CAD build for the part. Positions are in the model's coordinates, mm. A direction names the side the tool comes from. Coordinates: 2 decimals unless noted, no trailing zeros. Order: outer loops, then holes, each group sorted by start corner. A loop starts at its lowest first (then second) coordinate and runs counter-clockwise, first axis right, second up.
Autodesk Inventor part; units mm, degrees
ref_plane "Work Plane1" through (10.95, 0, 0) normal (0, 0, -1) x (1, 0, 0)
ref_plane "YZ Plane" through (0, 0, 0) normal (1, 0, 0) x (0, 1, 0)
ref_plane "XZ Plane" through (0, 0, 0) normal (0, 1, 0) x (-1, 0, 0)
sketch "Sketch1" plane through (0, 0, 0) normal (0, 0, 1) x (1, 0, 0)
  line L0 (-3.06, 0) -> (-3.06, 4.0996)
  line L1 (0, 5.7) -> (0, 3)
  line L2 (7, 3) -> (25, 3)
  line L3 (25, 3) -> (25, 0)
  line L4 (25, 0) -> (-3.06, 0)
  arc A0 (0, 5.7) -> (-2.0969, 6.1649) centre (-1.1, 5.7) ccw
  line L5 (0, -1.4013) -> (0, 8.4076)
  line L6 (-9.672, 0) -> (36.612, 0)
  line L7 (0, 3) -> (0.0001, 3)
  line L8 (0.0001, 3) -> (0.0001, 3)
  line L9 (0.0001, 3) -> (6.3865, 3)
  line L10 (6.3865, 3) -> (7, 3)
  line L11 (-3.06, 4.0996) -> (-2.0969, 6.1649)
  line L12 (0.0001, 3) -> (7, 3) construction
  line L13 (7, 3) -> (7, 0) construction
  dimension "d0" = 1.1
  dimension "d1" = 25
  dimension "d2" = 18
  dimension "d3" = 13.6
  dimension "d4" = 6
  dimension "d5" = 3.06
  dimension "d15" = 6
  dimension "d16" = 6
  dimension "d17" = 0.0001
  dimension "d18" = 0.6135
  dimension "d19" = 25
revolve "Body" add sketch "Sketch1" angle 360 about axis through (25, 0, 0) along (-1, 0, 0)
sketch "Sketch2" plane through (0, 0, 0) normal (1, 0, 0) x (0, 0, -1)
  line L0 (4, 2.3094) -> (4, -2.3094)
  line L1 (4, -2.3094) -> (0, -4.6188)
  line L2 (0, -4.6188) -> (-4, -2.3094)
  line L3 (-4, -2.3094) -> (-4, 2.3094)
  line L4 (-4, 2.3094) -> (0, 4.6188)
  line L5 (0, 4.6188) -> (4, 2.3094)
  point P0 (0, 0)
  point P1 (0, 0)
  dimension "d23" = 8
extrude "Head" add sketch "Sketch2" against normal blind 6.8
sketch "Sketch3" plane through (0, 0, 0) normal (0, 0, 1) x (1, 0, 0)
  line L0 (-6.8, 3.8) -> (-6.8, 4.6188)
  line L1 (-6.8, 4.6188) -> (-6.3273, 4.6188)
  line L2 (-6.3273, 4.6188) -> (-6.8, 3.8)
  line L3 (-7.5964, 0) -> (-2.0215, 0)
  line L4 (-6.8, 4.6188) -> (-6.8, 2.3094)
  line L5 (-2.8179, 4.6188) -> (-6.8, 4.6188)
  point P0 (-6.8, 2.3094)
  dimension "d8" = 30
  dimension "d22" = 7.6
revolve "Chamfer1" cut sketch "Sketch3" angle 360 about axis through (-10, 0, 0) along (1, 0, 0)
thread "Thread"
chamfer "Chamfer2" distance 0.6135 distance2 0.6135 1 edges at (25, -3, 0) measured on face at (25, -0.9709, -0.2393)
ref_plane "Work Plane1" through (10.95, 0, 0) normal (0, 0, -1) x (1, 0, 0)
equation "\"d0\" = PHH"
equation "\"d1\" = NLG"
equation "\"d2\" = GEL"
equation "\"d3\" = LADI"
equation "\"d4\" = GD"
equation "\"d5\" = 0.45 * KOH"
equation "\"d15\" = SD2"
equation "\"d16\" = BDM"
equation "\"d18\" = GAL"
equation "\"d19\" = KEWI"
equation "\"d23\" = SW"
equation "\"d6\" = KOH"
equation "\"d8\" = ANG1"
equation "\"d22\" = SW0"
equation "\"d10\" = GEL"
equation "\"d13\" = -0.5 * SPD + 0.5 * GD"
equation "\"d14\" = GUL"
equation "\"NLG\" = 25"
equation "\"GD\" = NND"
equation "\"BDM\" = NND"
equation "\"KOH\" = 6.8"
equation "\"GEL\" = 18"
equation "\"LADI\" = 13.6"
equation "\"SW\" = 8"
equation "\"PHH\" = RR"
equation "\"SW0\" = 7.6"
equation "\"SPD\" = NND - 1.2269 * PTC"
equation "\"SD2\" = NND"
equation "\"SD\" = 0"
equation "\"ANG1\" = 30deg"
equation "\"KEWI\" = 25deg"
equation "\"GAL\" = 0.61345 * PTC"
equation "\"GUL\" = 0.61345 * PTC"
equation "\"PTC\" = 1"
equation "\"THREADDIA\" = 6"
equation "\"E0\" = 1.155 * SW"
equation "\"TOA\" = 30deg"
equation "\"NND\" = 6"
equation "\"GD1\" = THREADDIA - 1.2269 * PTC"
equation "\"SDH\" = SW"
equation "\"KOH1\" = 2.9"
equation "\"RR\" = 1.1"
properties part number "ISO 4162 - M6 x 30" material "Stainless Steel"
1) Slice it at B-B (x = 4). List the corners of the cut face in (y, z), plus the area to 3 significant figures.
2) Slice it at A-A (y = 0). List the corners of the cut face in (x, z).
3) Pin check, flat tips, straight feed: P1, Ø4, axis at x = 1, y = -3.5, coming from the -Z side; P2, Ø3, axis at x = 11, y = -1.5, coming from the -Z side; P3, Ø5, axis at x = -2.5, y = -5, coming from the +Z side. Stop position of each tip, or through.
4) Which spindle directions (+Z, -Z, +X, -X, +Y, -Y) get a long thin tool onto all of the face, cutting with end or side? Do faces 4 (the flat face through (-4.72, -3.48, 1.97)), 5 (the flat face through (-6.8, 0, 0)), 6 (the flat face through (25, 0, 0)), 7 (the flat face through (-4.724, -3.448, -2.028)), 8 (the flat face through (-4.72, 3.48, -1.97)). Say none if no direction does.
5) Two-plate mould, pull along Y, no slides. Class faces 1 (the flat face through (-4.724, 3.448, 2.028)), 2 (the cylindrical face through (12, -3, 0)), 3 (the flat face through (0, 2.5, 2.5)): released by +Y, released by -Y, zero draft, split by the parting line, or undercut.
6) Drill centre lines: probe 1 along Z at (x, y) = (-4.5, -0.5); probe 2 along X at (y, z) = (-2.75, 5); probe 3 along X at (y, z) = (0.75, -3.5). Where is each one in solid material? Low to high.
Worked out:
1. outline: circle Ø6 at (0, 0)
1. area: 28.3 mm2
2. outline: (-6.8, -3.8) - (-6.68, -4) - (-3.06, -4) - (-3.06, -4.1) - (-2.1, -6.16) arc R1.1 ccw to (0, -5.7) - (0, -3) - (24.39, -3) - (25, -2.39) - (25, 2.39) - (24.39, 3) - (0, 3) - (0, 5.7) arc R1.1 ccw to (-2.1, 6.16) - (-3.06, 4.1) - (-3.06, 4) - (-6.68, 4) - (-6.8, 3.8) - close
3. P1: stops at z = -6.27
3. P2: stops at z = -3
3. P3: stops at z = 6.17
4. face 4: +Z, -X, -Y
4. face 5: +Z, -Z, -X, +Y, -Y
4. face 6: +Z, -Z, +X, +Y, -Y
4. face 7: -Z, -X, -Y
4. face 8: -Z, -X, +Y
5. face 1: released by +Y
5. face 2: split by the parting line
5. face 3: zero draft
6. probe 1: z = -4 to 4
6. probe 2: x = -2.31 to 0
6. probe 3: x = -6.8 to 0
